The model under review builds one solid part; all positions refer to its coordinate system, in mm. A direction names the side the tool comes from. Round coordinates to 2 decimals unless told otherwise and drop trailing zeros. Return JSON: item names as keys, results as strings. Group by question number.
Q1. For faces 1 (the face through (50.8, 1, 0)), 2 (the face through (-1, 1, 0)), list the 3-axis set-ups (+Z, -Z, +X, -X, +Y, -Y) from which the entire face can be reached by the end or side of a thin tool; tool diameter is ignored.
Q2. To check wall thickness, follow line 1 along Z through (x, y) = (-5, 17); line 2 along X through (y, z) = (7, -0.5); line 3 along X through (y, z) = (44.5, -0.7). State the ranges of each line that lie inside material, in increasing order.
Q3. Draft analysis for pull direction X (two halves, no side actions). For faces 3 (the face through (43.1, -43.2, -0.2)), 4 (the face through (-43.1, 43.2, -0.2)), 5 (the face through (46.98, 47.18, 0.02)), 6 (the face through (-43.51, 43.31, 2.34)), state which applies: pulls with the +X half, pulls with the -X half, needs draft (parallel to the pull), parting line crosses it, or undercut.
Q4. Clearance check with a flat-ended pin moving along its axis: pin 1 Ø8 at (x, y) = (-1.5, 4.5) entering from -Z. State where the tip first meets the part, or that it passes through.
from build123d import *

# Parameters (mm, degrees)
F1_DEPTH = 2.54
F3_DEPTH = 1.27
F5_DEPTH = 1.27
F6_SIZE  = 1.26999
F7_SIZE  = 1.26999


# Not quite as in the source:
# - a fillet or chamfer is up to 0.001 mm smaller than in the source, because OpenCascade refuses the exact size


with BuildPart() as f1:
    # F0 (on Top) → F1 (new body)
    with BuildSketch(Plane.XY):
        with BuildLine():
            ThreePointArc((50.8, 38.1), (47.0802561211, 47.0802561211), (38.1, 50.8))
            Line((38.1, 50.8), (-38.1, 50.8))
            ThreePointArc((-38.1, 50.8), (-47.0802561211, 47.0802561211), (-50.8, 38.1))
            Line((-50.8, 38.1), (-50.8, -38.1))
            ThreePointArc((-50.8, -38.1), (-47.0802561211, -47.0802561211), (-38.1, -50.8))
            Line((-38.1, -50.8), (38.1, -50.8))
            ThreePointArc((38.1, -50.8), (47.0802561211, -47.0802561211), (50.8, -38.1))
            Line((50.8, -38.1), (50.8, 38.1))
        make_face()
    extrude(amount=F1_DEPTH)

    # F2 (on face) → F3 (join)
    with BuildSketch(Plane(origin=(0, 0, 0), x_dir=(1, 0, 0), z_dir=(0, 0, -1))):
        with BuildLine():
            Line((-38.1, -50.8), (38.1, -50.8))
            ThreePointArc((38.1, -50.8), (47.0802561211, -47.0802561211), (50.8, -38.1))
            Line((50.8, -38.1), (50.8, 38.1))
            ThreePointArc((50.8, 38.1), (47.0802561211, 47.0802561211), (38.1, 50.8))
            Line((38.1, 50.8), (-38.1, 50.8))
            ThreePointArc((-38.1, 50.8), (-47.0802561211, 47.0802561211), (-50.8, 38.1))
            Line((-50.8, 38.1), (-50.8, -38.1))
            ThreePointArc((-50.8, -38.1), (-47.0802561211, -47.0802561211), (-38.1, -50.8))
        make_face()
        with BuildLine():
            Line((-34.925, 47.625), (34.925, 47.625))
            ThreePointArc((34.925, 47.625), (43.9052561211, 43.9052561211), (47.625, 34.925))
            Line((47.625, 34.925), (47.625, -34.925))
            ThreePointArc((47.625, -34.925), (43.9052561211, -43.9052561211), (34.925, -47.625))
            Line((34.925, -47.625), (-34.925, -47.625))
            ThreePointArc((-34.925, -47.625), (-43.9052561211, -43.9052561211), (-47.625, -34.925))
            Line((-47.625, -34.925), (-47.625, 34.925))
            ThreePointArc((-47.625, 34.925), (-43.9052561211, 43.9052561211), (-34.925, 47.625))
        make_face(mode=Mode.SUBTRACT)
    extrude(amount=F3_DEPTH)

    # F4 (on face) → F5 (cut)
    with BuildSketch(Plane.XY.offset(2.54)):
        with BuildLine():
            Line((50.8, -38.1), (50.8, 38.1))
            ThreePointArc((50.8, 38.1), (47.0802561211, 47.0802561211), (38.1, 50.8))
            Line((38.1, 50.8), (-38.1, 50.8))
            ThreePointArc((-38.1, 50.8), (-47.0802561211, 47.0802561211), (-50.8, 38.1))
            Line((-50.8, 38.1), (-50.8, -38.1))
            ThreePointArc((-50.8, -38.1), (-47.0802561211, -47.0802561211), (-38.1, -50.8))
            Line((-38.1, -50.8), (38.1, -50.8))
            ThreePointArc((38.1, -50.8), (47.0802561211, -47.0802561211), (50.8, -38.1))
        make_face()
        with BuildLine():
            ThreePointArc((46.99, -34.29), (43.2702561211, -43.2702561211), (34.29, -46.99))
            Line((34.29, -46.99), (-34.29, -46.99))
            ThreePointArc((-34.29, -46.99), (-43.2702561211, -43.2702561211), (-46.99, -34.29))
            Line((-46.99, -34.29), (-46.99, 34.29))
            ThreePointArc((-46.99, 34.29), (-43.2702561211, 43.2702561211), (-34.29, 46.99))
            Line((-34.29, 46.99), (34.29, 46.99))
            ThreePointArc((34.29, 46.99), (43.2702561211, 43.2702561211), (46.99, 34.29))
            Line((46.99, 34.29), (46.99, -34.29))
        make_face(mode=Mode.SUBTRACT)
    extrude(amount=-F5_DEPTH, mode=Mode.SUBTRACT)

    # F6 (size 1.27 in the source; OpenCascade refuses exactly that, so slightly less here)
    f6_edges = [f1.edges().sort_by_distance(p)[0] for p in [
        (0, 46.99, 1.27),
        (-43.270256, 43.270256, 1.27),
        (-46.99, 0, 1.27),
        (-43.270256, -43.270256, 1.27),
    ]]
    chamfer(f6_edges, length=F6_SIZE)

    # F7 (size 1.27 in the source; OpenCascade refuses exactly that, so slightly less here)
    f7_edges = [f1.edges().sort_by_distance(p)[0] for p in [
        (-43.905256, -43.905256, 0),
        (-47.625, 0, 0),
        (-43.905256, 43.905256, 0),
        (0, 47.625, 0),
        (43.905256, 43.905256, 0),
        (47.625, 0, 0),
        (43.905256, -43.905256, 0),
        (0, -47.625, 0),
    ]]
    chamfer(f7_edges, length=F7_SIZE)


solid = f1.part
Values:
{
 "1": {"face 1": "+Z, -Z, +X, +Y, -Y", "face 2": "-Z"},
 "2": {"line 1": "z = 0 to 2.54", "line 2": "x = -50.8 to -46.86, 46.86 to 50.8", "line 3": "x = -49.07 to -42.37, 42.37 to 49.07"},
 "3": {"face 3": "undercut", "face 4": "undercut", "face 5": "pulls with the +X half", "face 6": "pulls with the -X half"},
 "4": {"pin 1": "stops at z = 0"}
}
